CAD build for the part. Positions are in the model's coordinates, mm. A direction names the side the tool comes from. Give positions to 0.01 mm unless a question says otherwise; leave off trailing zeros. Loops run counter-clockwise (first coordinate to the right, second up) from the corner with the lowest first, then second, coordinate; pieces in that order, holes last.
Item 1: Probe probe 1 along Y at (x, z) = (7.75, 81.2); probe 2 along Y at (x, z) = (7, 79); probe 3 along Z at (x, y) = (-13, 4.5). List the from-to ranges inside material, lowest first.
Item 2: Saw through at D-D on y = -10. Give the cut face in (x, z).
Item 3: Saw through at C-C on z = 24. Give the cut face in (x, y), plus the area to 3 significant figures.
Item 4: Which spindle directions (+Z, -Z, +X, -X, +Y, -Y) get a long thin tool onto all of the face, cutting with end or side? Do faces 1 (the cylindrical face through (-4.01, 18.06, 68.06)), 2 (the cylindrical face through (8.663, 14.614, 80.479)), 3 (the flat face through (0, 9.5, 97)). Say none if no direction does.
Item 5: Mould opens along X. For faces 4 (the cylindrical face through (-14.2, 10.9, 26.9)), 5 (the flat face through (0, 0, 0)), 6 (the conical face through (7.591, -13.217, 78.255)) say: released by +X, released by -X, zero draft, split by the parting line, or undercut.
Item 6: Saw through at A-A on y = 7. Give the cut face in (x, z), plus the area to 3 significant figures.
Item 7: Saw through at B-B on x = -11. Give the cut face in (y, z), plus the area to 3 significant figures.
Item 8: Drop flat-ended pins along their axis: P1, Ø6, axis at y = -4.5, z = 71, coming from the -X side; P2, Ø18.5, axis at x = -7.5, y = -5, coming from the +Z side; P3, Ø6, axis at x = 9, z = 19, coming from the +Y side. Give the stop position or say it passes through.
Autodesk Inventor part; units mm, degrees
ref_plane "YZ Plane" through (0, 0, 0) normal (1, 0, 0) x (0, 1, 0)
ref_plane "XZ Plane" through (0, 0, 0) normal (0, 1, 0) x (-1, 0, 0)
ref_plane "XY Plane" through (0, 0, 0) normal (0, 0, 1) x (1, 0, 0)
sketch "スケッチ1" plane through (0, 0, 0) normal (0, 0, 1) x (1, 0, 0)
  circle A0 centre (0, 0) radius 17.9
  dimension "d0" = 35.8
extrude "押し出し1" add sketch "スケッチ1" along normal blind 54.5
sketch "スケッチ2" plane through (0, 0, 54.5) normal (0, 0, 1) x (1, 0, 0)
  circle A0 centre (0, 0) radius 17.9
  circle A1 centre (0, 0) radius 18.5
  dimension "d3" = 37
extrude "押し出し2" add sketch "スケッチ2" along normal blind 27.5 contours A0 | A1
sketch "スケッチ3" plane through (0, 0, 82) normal (0, 0, 1) x (1, 0, 0)
  circle A0 centre (0, 0) radius 18.5
  line L0 (0, 0) -> (0, 7)
  circle A1 centre (0, 7) radius 6
  dimension "d6" = 7
  dimension "d7" = 12
extrude "押し出し3" add sketch "スケッチ3" along normal blind 6 contours A1
sketch "スケッチ4" plane through (0, 7, 88) normal (0, 0, 1) x (1, 0, 0)
  circle A0 centre (0, 0) radius 6
  circle A1 centre (0, 0) radius 3
  point P0 (0, -7)
  dimension "d10" = 6
extrude "押し出し4" add sketch "スケッチ4" along normal blind 15 contours A1
sketch "スケッチ5" plane through (0, 7, 103) normal (0, 0, 1) x (1, 0, 0)
  circle A0 centre (0, 0) radius 3
  line L0 (0, -3) -> (0, 2.5)
  line L1 (0, 2.5) -> (1.6583, 2.5)
  line L2 (-1.6583, 2.5) -> (0, 2.5)
  point P0 (0, -7)
  dimension "d13" = 5.5
extrude "押し出し5" cut sketch "スケッチ5" against normal blind 12 contours L1 L2 A0
sketch "スケッチ6" plane through (0, 0, 82) normal (0, 0, 1) x (1, 0, 0)
  circle A0 centre (0, 0) radius 18.5
  circle A1 centre (0, 0) radius 15.5
  circle A2 centre (-15.5, 0) radius 1.5
  line L0 (0, 0) -> (7.75, 13.4234)
  line L1 (0, 0) -> (15.5, 0) construction
  line L2 (0, 0) -> (7.75, -13.4234)
  circle A3 centre (7.75, 13.4234) radius 1.5
  circle A4 centre (7.75, -13.4234) radius 1.5
  dimension "d16" = 31
  dimension "d17" = 3
  dimension "d18" = 60
  dimension "d19" = 3
  dimension "d20" = 3
hole "穴1" at (7.75, 13.4234, 82) at (-15.5, 0, 82) at (7.75, -13.4234, 82) direction (0, 0, -1) diameter 3 depth 3 tip angle 118
thread "ねじ1"
thread "ねじ2"
thread "ねじ3"
properties part number "知能ロボコンタミヤギヤードモータ540" material "鋼、炭素鋼"
Results below:
1. probe 1: y = -16.8 to -14.92, -11.92 to 11.92, 14.92 to 16.8
1. probe 2: y = -17.12 to -14.72, -12.12 to 12.12, 14.72 to 17.12
1. probe 3: z = 0 to 82
2. outline: (-15.56, 54.5) - (-14.85, 54.5) - (-14.85, 0) - (14.85, 0) - (14.85, 54.5) - (15.56, 54.5) - (15.56, 82) - (-15.56, 82) - close
3. outline: circle Ø35.8 at (0, 0)
3. area: 1,010 mm2
4. face 1: +Z, -Z
4. face 2: +Z
4. face 3: +Z, +X, -X, +Y
5. face 4: split by the parting line
5. face 5: zero draft
5. face 6: undercut
6. outline: (-17.12, 54.5) - (-16.47, 54.5) - (-16.47, 0) - (16.47, 0) - (16.47, 54.5) - (17.12, 54.5) - (17.12, 82) - (6, 82) - (6, 88) - (3, 88) - (3, 103) - (-3, 103) - (-3, 88) - (-6, 88) - (-6, 82) - (-17.12, 82) - close
6. area: 2,900 mm2
7. outline: (-14.87, 54.5) - (-14.12, 54.5) - (-14.12, 0) - (14.12, 0) - (14.12, 54.5) - (14.87, 54.5) - (14.87, 82) - (-14.87, 82) - close
7. area: 2,360 mm2
8. P1: stops at x = -18.44
8. P2: stops at z = 88
8. P3: stops at y = 16.86
